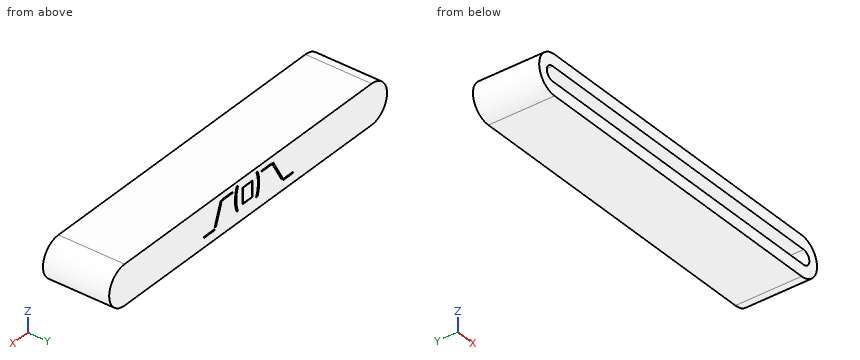
```python
from build123d import *

# Parameters (mm, degrees)
BOSS_EXTRUDE1_DEPTH = 12.7
CUT_EXTRUDE1_DEPTH  = 10.16
SKETCH3_W           = 2.512820512
SKETCH3_H           = 0.224358975
SKETCH3_W_2         = 2.512820513
SKETCH3_H_2         = 0.224358974
SKETCH3_W_3         = 2.423076923
SKETCH3_H_3         = 3.051282052
SKETCH3_W_4         = 2.243589743
SKETCH3_H_4         = 2.871794872
CUT_EXTRUDE2_DEPTH  = 1.27


with BuildPart() as part:
    # Sketch1 → Boss-Extrude1 (new body)
    with BuildSketch(Plane(origin=(0, 0, 0), x_dir=(1, 0, 0), z_dir=(0, 1, 0))):
        with BuildLine():
            Line((-30.48, 3.81), (30.48, 3.81))
            ThreePointArc((30.48, 3.81), (34.29, 0), (30.48, -3.81))
            Line((30.48, -3.81), (-30.48, -3.81))
            ThreePointArc((-30.48, -3.81), (-34.29, 0), (-30.48, 3.81))
        make_face()
    extrude(amount=BOSS_EXTRUDE1_DEPTH)

    # Sketch2 → Cut-Extrude1 (cut)
    with BuildSketch(Plane.XZ):
        with BuildLine():
            Line((-30.988, 1.397), (30.988, 1.397))
            ThreePointArc((30.988, 1.397), (32.385, 0), (30.988, -1.397))
            Line((30.988, -1.397), (-30.988, -1.397))
            ThreePointArc((-30.988, -1.397), (-32.385, 0), (-30.988, 1.397))
        make_face()
    extrude(amount=-CUT_EXTRUDE1_DEPTH, mode=Mode.SUBTRACT)

    # Sketch3 → Cut-Extrude2 (cut)
    with BuildSketch(Plane(origin=(0, 12.7, 0), x_dir=(1, 0, 0), z_dir=(0, 1, 0))):
        with Locations((-9.868354695, 1.949821987)):
            Rectangle(SKETCH3_W, SKETCH3_H)
        Polygon((-8.167433221, 1.56841173), (-5.874764951, -2.514921603), (-6.22953258, -2.514921603), (-8.522200849, 1.56841173), align=None)
        with Locations((-4.528611106, -2.492485706)):
            Rectangle(SKETCH3_W_2, SKETCH3_H_2)
        with BuildLine():
            Line((-2.329893156, 1.613283525), (-1.926047003, 1.613283525))
            add(Edge.make_bspline(
                [(-1.926047003, 1.613283525), (-1.944595679, 1.573225506), (-1.982258533, 1.491888205), (-2.033440085, 1.365776004), (-2.08306669, 1.235347225), (-2.128016891, 1.099286858), (-2.172746394, 0.958938117), (-2.212892282, 0.813055443), (-2.251030023, 0.662573196), (-2.297658473, 0.455059227), (-2.346937221, 0.189956446), (-2.388844661, -0.13371939), (-2.414835709, -0.462309009), (-2.418031025, -0.683310365), (-2.419636746, -0.794368719)],
                knots=[0, 0, 0, 0, 0.000132414, 0.000268864, 0.000408202, 0.000550987, 0.000698673, 0.00085007, 0.001004813, 0.001164361, 0.001488072, 0.00181332, 0.002143114, 0.002476253, 0.002476253, 0.002476253, 0.002476253], degree=3))
            add(Edge.make_bspline(
                [(-2.419636746, -0.794368719), (-2.418174092, -0.896994356), (-2.415269461, -1.100794888), (-2.39555112, -1.403593934), (-2.361748279, -1.700924317), (-2.315161311, -1.990560634), (-2.257008203, -2.26887028), (-2.187308319, -2.531522985), (-2.109429056, -2.777644099), (-2.046451105, -2.932917324), (-2.015790592, -3.008511347)],
                knots=[0, 0, 0, 0, 0.000307872, 0.000611392, 0.00090987, 0.001205296, 0.001491175, 0.001762426, 0.002020291, 0.002264936, 0.002264936, 0.002264936, 0.002264936], degree=3))
            Line((-2.015790592, -3.008511347), (-2.329893156, -3.008511347))
            add(Edge.make_bspline(
                [(-2.329893156, -3.008511347), (-2.345059433, -2.972840264), (-2.375799242, -2.900540233), (-2.418668441, -2.788874123), (-2.458438817, -2.672275035), (-2.496197017, -2.551137941), (-2.531986826, -2.425372334), (-2.565708096, -2.295224557), (-2.596352522, -2.160231418), (-2.635037976, -1.973771045), (-2.674487586, -1.734133797), (-2.708879678, -1.441012576), (-2.729583163, -1.141957485), (-2.732346302, -0.940701584), (-2.73373931, -0.839240513)],
                knots=[0, 0, 0, 0, 0.000116278, 0.000235679, 0.000358736, 0.000485801, 0.000616297, 0.000750978, 0.000889083, 0.001031536, 0.001322232, 0.001617307, 0.001916676, 0.002221044, 0.002221044, 0.002221044, 0.002221044], degree=3))
            add(Edge.make_bspline(
                [(-2.73373931, -0.839240513), (-2.732594304, -0.729601973), (-2.730314646, -0.511316432), (-2.709927037, -0.186438945), (-2.67775989, 0.134220277), (-2.63330287, 0.449137671), (-2.576047932, 0.75631684), (-2.506720854, 1.052993625), (-2.425998034, 1.33841465), (-2.36165775, 1.522433838), (-2.329893156, 1.613283525)],
                knots=[0, 0, 0, 0, 0.000328887, 0.000654799, 0.000976133, 0.001295507, 0.001608623, 0.001913212, 0.002209258, 0.002497933, 0.002497933, 0.002497933, 0.002497933], degree=3))
        make_face()
        with Locations((0.182927357, -0.495690834)):
            Rectangle(SKETCH3_W_3, SKETCH3_H_3)
        with Locations((0.182927357, -0.495690834)):
            Rectangle(SKETCH3_W_4, SKETCH3_H_4, mode=Mode.SUBTRACT)
        with BuildLine():
            Line((2.830363254, -3.008511347), (2.4265171, -3.008511347))
            add(Edge.make_bspline(
                [(2.4265171, -3.008511347), (2.445363004, -2.968481706), (2.483586773, -2.887292514), (2.534455272, -2.76084909), (2.584889971, -2.630579527), (2.630978179, -2.494786752), (2.674142382, -2.354187151), (2.715314887, -2.208721317), (2.751721509, -2.058090142), (2.799164465, -1.850839452), (2.848318586, -1.585696239), (2.889036553, -1.261679417), (2.915372484, -0.932926529), (2.918523423, -0.711920038), (2.920106844, -0.600859103)],
                knots=[0, 0, 0, 0, 0.000132705, 0.000269155, 0.000408742, 0.000551752, 0.000699229, 0.000849951, 0.001005205, 0.001164069, 0.001487781, 0.001813634, 0.002143428, 0.002476567, 0.002476567, 0.002476567, 0.002476567], degree=3))
            add(Edge.make_bspline(
                [(2.920106844, -0.600859103), (2.918636197, -0.498001444), (2.91572232, -0.294203706), (2.896183473, 0.008881128), (2.861380724, 0.305887024), (2.815003035, 0.595585979), (2.756388988, 0.873712258), (2.688249953, 1.13672272), (2.609689621, 1.382585825), (2.546879933, 1.537677511), (2.51626069, 1.613283525)],
                knots=[0, 0, 0, 0, 0.000308573, 0.000611394, 0.000910648, 0.001205381, 0.001491261, 0.001763011, 0.002020209, 0.002264854, 0.002264854, 0.002264854, 0.002264854], degree=3))
            Line((2.51626069, 1.613283525), (2.830363254, 1.613283525))
            add(Edge.make_bspline(
                [(2.830363254, 1.613283525), (2.845822151, 1.577637011), (2.877117965, 1.505472313), (2.919829121, 1.393322705), (2.960040307, 1.276737462), (2.999155723, 1.155636367), (3.034577994, 1.029732856), (3.067427606, 0.898965664), (3.098479857, 0.763700098), (3.135574411, 0.576263016), (3.175988281, 0.336649903), (3.209135848, 0.043155631), (3.230099589, -0.255833632), (3.232832988, -0.457328041), (3.234209408, -0.558791796)],
                knots=[0, 0, 0, 0, 0.000116551, 0.000235952, 0.0003599, 0.000486508, 0.000617678, 0.000752185, 0.000890974, 0.001033975, 0.001325362, 0.00161966, 0.001919729, 0.002224096, 0.002224096, 0.002224096, 0.002224096], degree=3))
            add(Edge.make_bspline(
                [(3.234209408, -0.558791796), (3.233086955, -0.66819864), (3.230857007, -0.885554545), (3.210174372, -1.209702469), (3.178588831, -1.529761994), (3.132817504, -1.84453593), (3.075650132, -2.151444658), (3.007392512, -2.448324515), (2.926416312, -2.733629989), (2.86211072, -2.917657534), (2.830363254, -3.008511347)],
                knots=[0, 0, 0, 0, 0.000328186, 0.000651998, 0.00097403, 0.001292809, 0.001605925, 0.001910355, 0.002206401, 0.002495076, 0.002495076, 0.002495076, 0.002495076], degree=3))
        make_face()
        with Locations((5.073952998, -2.492485706)):
            Rectangle(SKETCH3_W_2, SKETCH3_H_2)
        Polygon((8.259850433, 1.56841173), (6.795908126, -2.514921603), (6.464978638, -2.514921603), (7.928920946, 1.56841173), align=None)
        with Locations((9.60600428, 1.949821987)):
            Rectangle(SKETCH3_W_2, SKETCH3_H)
    extrude(amount=-CUT_EXTRUDE2_DEPTH, mode=Mode.SUBTRACT)


solid = part.part
```
Here's how the part is built. I have some questions about the finished solid (model axes, mm). Coordinates: 2 decimals unless noted, no trailing zeros. Order: outer loops, then holes, each group sorted by start corner. A loop starts at its lowest first (then second) coordinate and runs counter-clockwise, first axis right, second up.
1) I need wall thicknesses on line 1 (Z direction, x = -24, y = 8.75); line 2 (X direction, y = 8, z = 0) (3 decimals); line 3 (Y direction, x = -28, z = 0.25). Which ranges of each line are inside material? Lowest first, please.
2) Imagine slicing it at B-B on x = -14.5. List the corners of the cut face in (y, z) for me, and give its area (3 significant figures).
3) Imagine slicing it at A-A on y = 4.75. List the corners of the cut face in (x, z) for me, and give its area (3 significant figures).
Response values:
1. line 1: z = -3.81 to -1.4, 1.4 to 3.81
1. line 2: x = -34.29 to -32.385, 32.385 to 34.29
1. line 3: y = 10.16 to 12.7
2. outline: (0, -3.81) - (12.7, -3.81) - (12.7, 3.81) - (0, 3.81) - (0, 1.4) - (10.16, 1.4) - (10.16, -1.4) - (0, -1.4) - close
2. area: 68.4 mm2
3. outline: (-30.48, -3.81) - (30.48, -3.81) arc R3.81 ccw to (30.48, 3.81) - (-30.48, 3.81) arc R3.81 ccw to start; hole (-30.99, -1.4) - (30.99, -1.4) arc R1.4 ccw to (30.99, 1.4) - (-30.99, 1.4) arc R1.4 ccw to start
3. area: 331 mm2
